Build history of the part. All positions in model axes, mm. A direction names the side the tool comes from. Coordinates: 2 decimals unless noted, no trailing zeros. Order: outer loops, then holes, each group sorted by start corner. A loop starts at its lowest first (then second) coordinate and runs counter-clockwise, first axis right, second up. Notation, with made-up numbers: (79.5, -37.5) - (138.5, -37.5) arc R16 cw to (138.5, -26.5) - close; hole circle Ø1 at (-32.5, 19.5). An arc over 180 degrees is marked (long way). One line per item, written item: value.
Autodesk Inventor part; units mm, degrees
ref_plane "YZ Plane" through (0, 0, 0) normal (1, 0, 0) x (0, 1, 0)
ref_plane "XZ Plane" through (0, 0, 0) normal (0, 1, 0) x (-1, 0, 0)
ref_plane "XY Plane" through (0, 0, 0) normal (0, 0, 1) x (1, 0, 0)
sketch "Sketch1" plane through (0, 0, 0) normal (0, 1, 0) x (-1, 0, 0)
  line L0 (0, 0) -> (284.48, 0)
  line L1 (284.48, 0) -> (284.48, 106.68)
  line L2 (284.48, 106.68) -> (0, 106.68)
  line L3 (0, 106.68) -> (0, 0)
  line L4 (0, 53.34) -> (27.305, 53.34) construction
  line L5 (284.48, 53.34) -> (257.175, 53.34) construction
  circle A0 centre (27.305, 53.34) radius 12.7
  circle A1 centre (257.175, 53.34) radius 12.7
  dimension "d0" = 284.48
  dimension "d1" = 106.68
  dimension "d2" = 27.305
  dimension "d3" = 27.305
  dimension "d4" = 25.4
  dimension "d5" = 25.4
extrude "Extrusion1" add sketch "Sketch1" along normal blind 20.32
sketch "Sketch2" plane through (0, 20.32, 0) normal (0, 1, 0) x (1, 0, 0)
  circle A0 centre (-257.175, -53.34) radius 12.7
  circle A1 centre (-27.305, -53.34) radius 12.7
  circle A2 centre (-257.175, -53.34) radius 22.86
  circle A3 centre (-27.305, -53.34) radius 22.86
  dimension "d8" = 45.72
  dimension "d9" = 45.72
extrude "Extrusion2" add sketch "Sketch2" along normal blind 20.32
sketch "Sketch3" plane through (-284.48, 0, 0) normal (-1, 0, 0) x (0, 0, 1)
  line L0 (0, 0) -> (106.68, 0)
  line L1 (106.68, 0) -> (106.68, 20.32)
  line L2 (0, 20.32) -> (106.68, 20.32)
  line L3 (0, 0) -> (0, 20.32)
extrude "Extrusion3" add sketch "Sketch3" along normal blind 27.94
sketch "Sketch4" plane through (0, 0, 106.68) normal (1, 0, 0) x (0, 0, -1)
  line L0 (0, 0) -> (106.68, 0)
  line L1 (106.68, 0) -> (106.68, 20.32)
  line L2 (0, 20.32) -> (106.68, 20.32)
  line L3 (0, 0) -> (0, 20.32)
extrude "Extrusion4" add sketch "Sketch4" along normal blind 27.94
fillet "Fillet1" radius 1 13 edges at (-312.42, 10.16, 106.68) (-142.24, 0, 106.68) (-142.24, 0, 0) (-312.42, 0, 53.34) (27.94, 0, 53.34) (27.94, 10.16, 106.68) (27.94, 10.16, 0) (-142.24, 20.32, 0) (27.94, 20.32, 53.34) (-142.24, 20.32, 106.68) (-312.42, 20.32, 53.34) (-280.035, 40.64, 53.34) (-50.165, 40.64, 53.34)
equation "\"d2\" = d3"
properties part number "CIM MountBase" material "Aluminum 6061, Welded"
1. Band-saw the part on C-C, the plane z = 16. Give the cut face in (x, y).
Values found:
outline: (-312.42, 1) arc R1 ccw to (-311.42, 0) - (26.94, 0) arc R1 ccw to (27.94, 1) - (27.94, 19.32) arc R1 ccw to (26.94, 20.32) - (-311.42, 20.32) arc R1 ccw to (-312.42, 19.32) - close
2. Band-saw the part on A-A, the plane y = 9. Give the cut face in (x, z) (3 decimals), and give its area (3 significant figures).
Values found:
outline: (-312.42, 0) - (26.94, 0) arc R1 ccw to (27.94, 1) - (27.94, 105.68) arc R1 ccw to (26.94, 106.68) - (-311.42, 106.68) arc R1 ccw to (-312.42, 105.68) - close; hole circle Ø25.4 at (-257.175, 53.34); hole circle Ø25.4 at (-27.305, 53.34)
area: 35,300 mm2
3. Probe line 1 along X through (y, z) = (15, 53); line 2 along X through (y, z) = (32, 53); line 3 along X through (y, z) = (29, 53.34) (3 decimals). List the from-to ranges inside material, lowest first.
Values found:
line 1: x = -312.42 to -269.87, -244.48 to -40, -14.61 to 27.94
line 2: x = -280.03 to -269.87, -244.48 to -234.32, -50.16 to -40, -14.61 to -4.45
line 3: x = -280.035 to -269.875, -244.475 to -234.315, -50.165 to -40.005, -14.605 to -4.445
4. Flat gauge pins, fed straight in: P1, Ø1, axis at x = -245, y = 35.5, coming from the +Z side; P2, Ø4, axis at x = -118.5, z = 62, coming from the +Y side; P3, Ø10, axis at x = -200, y = 4, coming from the -Z side. Where does each tip first touch, or does it go through?
Values found:
P1: stops at z = 72.99
P2: stops at y = 20.32
P3: stops at z = 0
5. 3-axis set-ups, long thin cutter, end or side, ignore diameter. For faces 1 (the face through (-236.06, 29.84, 44.58)), 2 (the face through (-18, 40.64, 63)): which of +Z, -Z, +X, -X, +Y, -Y reach the whole face in a straight line?
Values found:
face 1: +Y
face 2: +Z, -Z, +X, -X, +Y
6. Band-saw the part on B-B, the plane y = 31. Give the cut face in (x, z) (3 decimals).
Values found:
outline: circle Ø45.72 at (-257.175, 53.34); circle Ø45.72 at (-27.305, 53.34); hole circle Ø25.4 at (-257.175, 53.34); hole circle Ø25.4 at (-27.305, 53.34)
